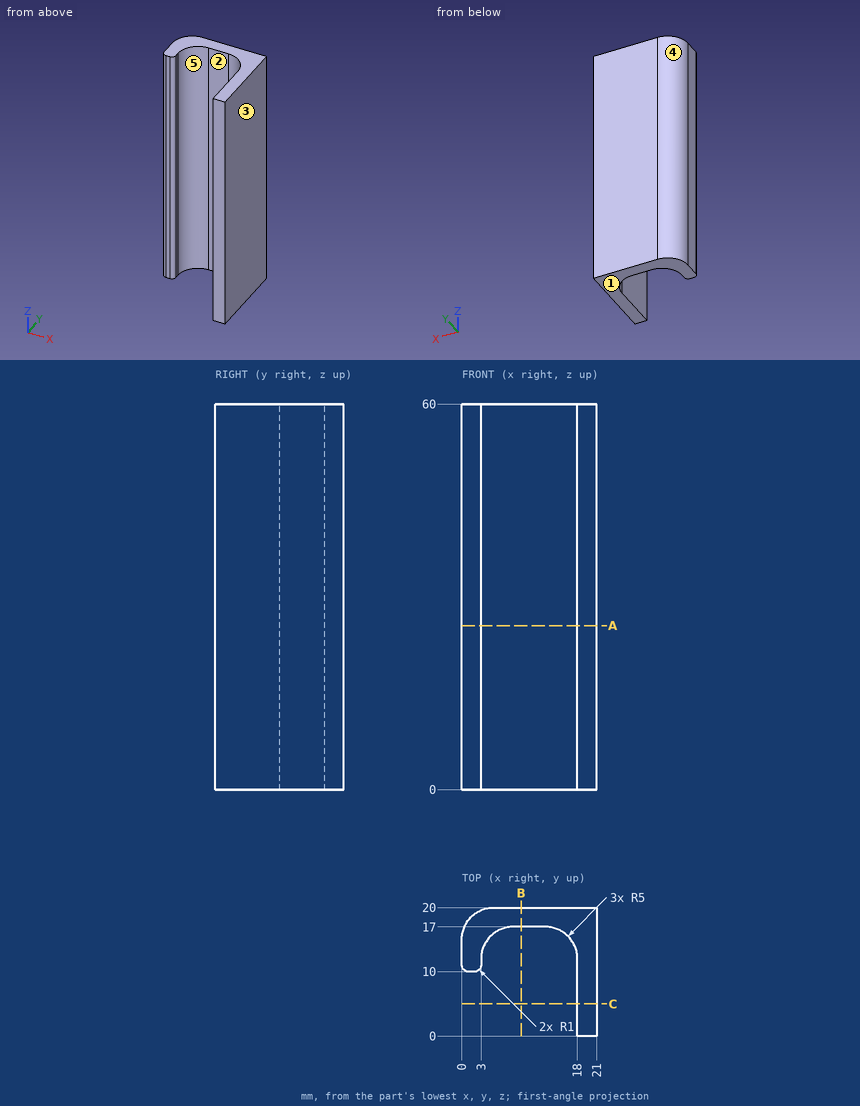
Study the drawing (mm; zero at the part's minimum x, y, z) and answer. A direction names the side the tool comes from. Round coordinates to 2 decimals unless told otherwise and drop trailing zeros. Loops run counter-clockwise (first coordinate to the right, second up) from the corner with the lowest first, then second, coordinate; pieces in that order, holes last. Notation, with made-up numbers: (34, 82.25) - (39, 82.25) arc R19 ccw to (39, 112.25) - close; hole circle Ø11 at (43, -39.75). An arc over 180 degrees is marked (long way). Use one line per item in the form item = value. Start each with the question number.
1. The part is cut by section B-B on x = 9.25. Determine the outline of the cut face in (y, z), then the cut area to 3 significant figures.
2. The part is cut by section C-C on y = 5. Determine the outline of the cut face in (x, z), then the cut area to 3 significant figures.
3. For a pull along X with two mould halves and no side action, classify the marked faces 3, 4 and 5 as pulls with the +X half, pulls with the -X half, needs draft (parallel to the pull), parting line crosses it, or undercut.
4. The part is cut by section A-A on z = 25.5. Determine the outline of the cut face in (x, y), then the cut area to 3 significant figures.
5. Consider line 1 (X direction, y = 12, z = 13.5); line 2 (X direction, y = 3, z = 4.5); line 3 (Y direction, x = 11, z = 28). Determine where each line is inside the solid, lowest interval first. Write a range as [from, to].
6. Given pin 1 Ø2.5 at (x, z) = (9.5, 22.5) entering from -Y; pin 2 Ø12 at (x, z) = (7, 53) entering from -Y; pin 3 Ø9.5 at (y, z) = (4, 15.5) entering from -X, each flat-ended and moving along its own axis, determine where each tip first touches the part or whether it passes through.
7. A tool of negligible diameter and unlimited length cuts with its end or side. For the marked faces 1 and 2, from which of +Z, -Z, +X, -X, +Y, -Y can it reach the whole face along a straight path? Write none if from no direction.
Geometry check:
q1.outline = (17, 0) - (20, 0) - (20, 60) - (17, 60) - close
q1.area = 180 mm^2
q2.outline = (18, 0) - (21, 0) - (21, 60) - (18, 60) - close
q2.area = 180 mm^2
q3.face_3 = pulls with the +X half
q3.face_4 = pulls with the -X half
q3.face_5 = undercut
q4.outline = (0, 11) arc R1 ccw to (1, 10) - (2, 10) arc R1 ccw to (3, 11) - (3, 12) arc R5 cw to (8, 17) - (13, 17) arc R5 cw to (18, 12) - (18, 0) - (21, 0) - (21, 20) - (5, 20) arc R5 ccw to (0, 15) - close
q4.area = 140 mm^2
q5.line_1 = [0, 3], [18, 21]
q5.line_2 = [18, 21]
q5.line_3 = [17, 20]
q6.pin_1 = 17
q6.pin_2 = 10
q6.pin_3 = 18
q7.face_1 = -Z, +X, -X, +Y, -Y
q7.face_2 = +Z, -Z, -Y
